Part model, mm, in its own coordinate system. A direction names the side the tool comes from. Round coordinates to 2 decimals unless told otherwise and drop trailing zeros. Order: outer loops, then holes, each group sorted by start corner. A loop starts at its lowest first (then second) coordinate and runs counter-clockwise, first axis right, second up. Notation, with made-up numbers: M 63,64.5 L 89,64.5 A19 cw 89,97.5 Z; hole C 81,4.5 d6. An arc over 180 degrees is marked long. Write each question's results on one line, items separated by ' | '. Start each with the question number.
1. Which spindle directions (+Z, -Z, +X, -X, +Y, -Y) get a long thin tool onto all of the face, cutting with end or side? Do faces 5 (the face through (165.1, -1, 87)), 6 (the face through (2, -1, 177.8)), 7 (the face through (52, 0, 307)), 8 (the face through (2, 88.9, 180)), 9 (the face through (-171.45, 21, 136)). Say none if no direction does.
2. Band-saw the part on D-D, the plane y = -22. List the corners of the cut face in (x, z), then the cut area to 3 significant figures.
3. Drop flat-ended pins along their axis: pin 1 Ø4 at (x, y) = (59, -19) entering from +Z; pin 2 Ø4 at (x, z) = (110, 97.5) entering from -Y. Give the stop position or say it passes through.
4. Two-plate mould, pull along Z, no slides. Class faces 1 (the face through (165.1, 41, 330)), 2 (the face through (77, 85, 0)), 3 (the face through (77, -82.55, 175)), 4 (the face through (2, 44, 355.6)): +Z half, -Z half, draft (parallel to the pull), parting line (faces both ways), or undercut.
5. Probe L1, parallel to Z at x = -123, y = 33; L2, parallel to X at y = 22, z = 60; L3, parallel to Y at x = 52.5, z = 17. List the from-to ranges inside material, lowest first. Write a range as [from, to].
6. Band-saw the part on C-C, the plane x = 130. List the corners of the cut face in (y, z).
7. Band-saw the part on B-B, the plane z = 293.5. List the corners of the cut face in (x, y), then the cut area to 3 significant figures.
8. Band-saw the part on A-A, the plane y = 9.5. List the corners of the cut face in (x, z).
```python
from build123d import *

# Parameters (mm, degrees)
F2_DEPTH = 6.35
F3_W     = 165.1
F3_H     = 6.35
F4_DEPTH = 165.1
F5_W     = 165.1
F5_H     = 6.35
F6_DEPTH = 82.55
F8_W     = 342.9
F8_H     = 355.6
F9_DEPTH = 6.35


with BuildPart() as f2:
    # F1 (on offset) → F2 (new body)
    with BuildSketch(Plane.YZ.offset(165.1)):
        Polygon((-82.55, 177.8), (-82.55, 0), (82.55, 0), (82.55, 355.6), (0, 355.6), (0, 177.8), align=None)
    extrude(amount=F2_DEPTH)

    # F3 (on face) → F4 (join, through all)
    with BuildSketch(Plane.XZ.offset(82.55)):
        with Locations((82.55, 174.625)):
            Rectangle(F3_W, F3_H)
    extrude(amount=-F4_DEPTH)

    # F5 (on face) → F6 (join, through all)
    with BuildSketch(Plane.XZ):
        with Locations((82.55, 352.425)):
            Rectangle(F5_W, F5_H)
        with Locations((82.55, 307.975)):
            Rectangle(F5_W, F5_H)
    extrude(amount=-F6_DEPTH)

    # F7: F2 across plane


with BuildPart() as f2_1:
    add(f2.part)
    add(f2.part.mirror(Plane.YZ))

    # F8 (on face) → F9 (join)
    with BuildSketch(Plane(origin=(0, 82.55, 0), x_dir=(-1, 0, 0), z_dir=(0, 1, 0))):
        with Locations((0, 177.8)):
            Rectangle(F8_W, F8_H)
    extrude(amount=F9_DEPTH)


solid = f2_1.part
```
Solution:
1) face 5: -Z, -Y | face 6: -Y | face 7: +Z, +X, -X, -Y | face 8: +Z, -Z, +X, -X, +Y | face 9: +Z, -Z, -X, +Y, -Y
2) outline: M -171.45,0 L -165.1,0 L -165.1,171.45 L 165.1,171.45 L 165.1,0 L 171.45,0 L 171.45,177.8 L -171.45,177.8 Z | area: 4,350 mm^2
3) pin 1: z = 177.8 | pin 2: y = 82.55
4) face 1: undercut | face 2: -Z half | face 3: draft | face 4: +Z half
5) L1: [171.45, 177.8], [304.8, 311.15], [349.25, 355.6] | L2: [-171.45, -165.1], [165.1, 171.45] | L3: [82.55, 88.9]
6) outline: M -82.55,171.45 L 82.55,171.45 L 82.55,0 L 88.9,0 L 88.9,355.6 L 0,355.6 L 0,349.25 L 82.55,349.25 L 82.55,311.15 L 0,311.15 L 0,304.8 L 82.55,304.8 L 82.55,177.8 L -82.55,177.8 Z
7) outline: M -171.45,0 L -165.1,0 L -165.1,82.55 L 165.1,82.55 L 165.1,0 L 171.45,0 L 171.45,88.9 L -171.45,88.9 Z | area: 3,230 mm^2
8) outline: M -171.45,0 L -165.1,0 L -165.1,171.45 L 165.1,171.45 L 165.1,0 L 171.45,0 L 171.45,355.6 L -171.45,355.6 Z; hole M -165.1,177.8 L 165.1,177.8 L 165.1,304.8 L -165.1,304.8 Z; hole M -165.1,311.15 L 165.1,311.15 L 165.1,349.25 L -165.1,349.25 Z
